Geometry check sheet. Reference: the model listing, model coordinates, mm. A direction names the side the tool comes from. Give positions to 0.01 mm unless a question says otherwise; leave off trailing zeros. Loops run counter-clockwise (first coordinate to the right, second up) from the corner with the lowest first, then second, coordinate; pieces in that order, holes last. Notation, with made-up numbers: (-5, 64.25) - (24, 64.25) arc R17 ccw to (24, 72.25) - close; hole circle Ø6 at (-17.5, 54). An arc over 180 degrees is marked (long way). Use a Markdown table: item, result. Add a question column.
1. Set-up check for faces 1 (the flat face through (0, 3, -16)), 2 (the cylindrical face through (-3.715, 1.521, 19.699)), 3 (the flat face through (0, 3, 16)): record each of +Z, -Z, +X, -X, +Y, -Y from which the full face is reachable in a straight line by a thin tool's end or side.
2. Cross-section at A-A on y = 0.8. Enter the section's corners in (x, z).
3. Cross-section at B-B on z = -13.5. Enter the section's corners in (x, y).
4. Material ranges on L1, parallel to Z at x = 0, y = 1.8; L2, parallel to X at y = 1.5, z = -13.5; L3, parallel to Z at x = 1.75, y = 1.75, recorded low to high.
5. Cross-section at D-D on z = 13. Enter the section's corners in (x, y), and give its area (3 significant figures).
6. Cross-section at C-C on x = 0. Count the separate pieces of the cut face and the enclosed holes in it, and give its area (3 significant figures).
7. Draft check along Z on faces 4 (the cylindrical face through (-3.699, 1.521, -19.715)), 5 (the cylindrical face through (3.699, 1.521, 19.715)), 6 (the cylindrical face through (-0.26, 1.521, -15.483)). Enter one of: pulls with the +Z half, pulls with the -Z half, needs draft (parallel to the pull), parting line crosses it, or undercut.
8. Depth check by flat-ended pin: P1, Ø4, axis at x = 1, z = -13, coming from the +Y side; P2, Ø3, axis at x = 0, z = -13.5, coming from the -Y side. Enter the tip coordinate at first touch or a pass-through.
Autodesk Inventor part; units mm, degrees
ref_plane "YZ Plane" through (0, 0, 0) normal (1, 0, 0) x (0, 1, 0)
ref_plane "XZ Plane" through (0, 0, 0) normal (0, 1, 0) x (-1, 0, 0)
ref_plane "XY Plane" through (0, 0, 0) normal (0, 0, 1) x (1, 0, 0)
sketch "Sketch1" plane through (0, 0, 0) normal (0, 1, 0) x (-1, 0, 0)
  line L0 (-4, 20) -> (4, 20)
  line L1 (4, 20) -> (4, -20)
  line L2 (4, -20) -> (-4, -20)
  line L3 (-4, -20) -> (-4, 20)
  line L4 (-4, 20) -> (4, -20) construction
  line L5 (4, 20) -> (-4, -20) construction
  point P0 (0, 0)
  dimension "d0" = 8
  dimension "d1" = 40
extrude "Extrusion1" add sketch "Sketch1" along normal blind 3
fillet "Fillet1" radius 1 4 edges at (4, 1.5, 20) (-4, 1.5, 20) (4, 1.5, -20) (-4, 1.5, -20)
sketch "Sketch2" plane through (0, 3, 0) normal (0, 1, 0) x (1, 0, 0)
  line L0 (0, 0) -> (0, -13.5) construction
  line L1 (0, 0) -> (0, 13.5) construction
  circle A0 centre (0, -13.5) radius 2
  circle A1 centre (0, 13.5) radius 2
  dimension "d5" = 13.5
  dimension "d6" = 13.5
  dimension "d7" = 4
  dimension "d8" = 4
extrude "Extrusion2" cut sketch "Sketch2" against normal up to surface (3 mm away)
sketch "Sketch3" plane through (0, 3, 0) normal (0, 1, 0) x (1, 0, 0)
  line L0 (-4, 9.5) -> (4, 9.5)
  line L1 (4, 9.5) -> (4, -9.5)
  line L2 (4, -9.5) -> (-4, -9.5)
  line L3 (-4, -9.5) -> (-4, 9.5)
  line L4 (-4, 9.5) -> (4, -9.5) construction
  line L5 (4, 9.5) -> (-4, -9.5) construction
  point P0 (0, 0)
  dimension "d11" = 8
  dimension "d12" = 19
extrude "Extrusion3" add sketch "Sketch3" along normal blind 1
chamfer "Chamfer1" distance 1 angle 45 4 edges at (0, 4, 9.5) (0, 4, -9.5) (4, 4, 0) (-4, 4, 0)
properties part number "load_cell"
Values found:
| question | item | result |
|---|---|---|
| 1 | face 1 | -Z, +X, -X, +Y |
| 1 | face 2 | +Z, -X, +Y, -Y |
| 1 | face 3 | +Z, +X, -X, +Y |
| 2 | outline | (-4, -19) arc R1 ccw to (-3, -20) - (3, -20) arc R1 ccw to (4, -19) - (4, 19) arc R1 ccw to (3, 20) - (-3, 20) arc R1 ccw to (-4, 19) - close; hole circle Ø4 at (0, -13.5); hole circle Ø4 at (0, 13.5) |
| 3 | outline | (-4, 0) - (-2, 0) - (-2, 3) - (-4, 3) - close; (2, 0) - (4, 0) - (4, 3) - (2, 3) - close |
| 4 | L1 | z = -20 to -15.5, -11.5 to 11.5, 15.5 to 20 |
| 4 | L2 | x = -4 to -2, 2 to 4 |
| 4 | L3 | z = -20 to -14.47, -12.53 to 12.53, 14.47 to 20 |
| 5 | outline | (-4, 0) - (-1.94, 0) - (-1.94, 3) - (-4, 3) - close; (1.94, 0) - (4, 0) - (4, 3) - (1.94, 3) - close |
| 5 | area | 12.4 mm2 |
| 6 | separate pieces | 3 |
| 6 | enclosed holes | 0 |
| 6 | area | 114 mm2 |
| 7 | face 4 | pulls with the -Z half |
| 7 | face 5 | pulls with the +Z half |
| 7 | face 6 | undercut |
| 8 | P1 | stops at y = 3 |
| 8 | P2 | passes through |
